Geometry check sheet. Reference: drawing and pictorial views, mm from the part's lowest x, y, z. Give positions to 0.01 mm unless a question says otherwise; leave off trailing zeros. Order: outer loops, then holes, each group sorted by start corner. A loop starts at its lowest first (then second) coordinate and runs counter-clockwise, first axis right, second up.
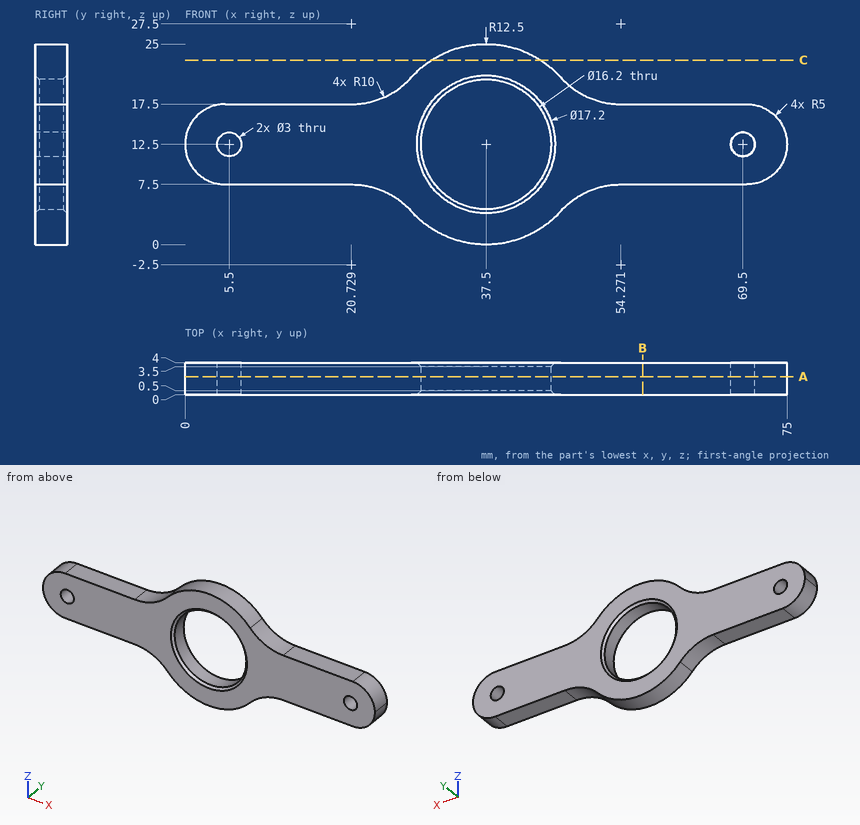
(1) Cross-section at B-B on x = 57. Enter the section's corners in (y, z).
Response values:
outline: (0, 7.5) - (4, 7.5) - (4, 17.5) - (0, 17.5) - close
(2) Cross-section at C-C on z = 23. Enter the section's corners in (x, y).
Response values:
outline: (30.72, 0) - (44.28, 0) - (44.28, 4) - (30.72, 4) - close
(3) Material ranges on L1, parallel to X at y = 1.6, z = 12.5; L2, parallel to Z at x = 56, y = 1.6; L3, parallel to Z at x = 42.5, y = 1.9 (1 decimal), recorded low to high.
Response values:
L1: x = 0 to 4, 7 to 29.4, 45.6 to 68, 71 to 75
L2: z = 7.5 to 17.5
L3: z = 1 to 6.1, 18.9 to 24
(4) Gauge pin test, flat ends, axial feed: pin 1 Ø1.2 at (x, y) = (13, 1.5) entering from -Z; pin 2 Ø1 at (x, y) = (28.5, 1) entering from +Z (1 decimal); pin 3 Ø1.2 at (x, y) = (66, 3) entering from +Z; pin 4 Ø2 at (x, z) = (42, 8) entering from -Y. Record the tip position at first contact, or that the pin passes through.
Response values:
pin 1: stops at z = 7.5
pin 2: stops at z = 21.7
pin 3: stops at z = 17.5
pin 4: passes through
(5) Cross-section at A-A on y = 2.25. Count the separate pieces of the cut face and the enclosed holes in it.
Response values:
separate pieces: 1
enclosed holes: 3
